from build123d import *

# Parameters (mm, degrees)
BOSS_EXTRUDE1_DEPTH      = 2.8
BOSS_EXTRUDE1_DEPTH_BACK = 2.8
ECHELLE1_SCALE           = 2
SKETCH2_R                = 1.55
CUT_EXTRUDE6_DEPTH       = 11.2


with BuildPart() as part:
    # Sketch1 → Boss-Extrude1 (new, two sides: drawn at the far end of the back side and taken through both)
    with BuildSketch(Plane.XY.offset(-BOSS_EXTRUDE1_DEPTH_BACK)):
        with BuildLine():
            Line((-33.309608541, 3.5), (9.690391459, 3.5))
            ThreePointArc((9.690391459, 3.5), (13.190391459, 0), (9.690391459, -3.5))
            Line((9.690391459, -3.5), (-33.309608541, -3.5))
            ThreePointArc((-33.309608541, -3.5), (-36.809608541, 0), (-33.309608541, 3.5))
        make_face()
    extrude(amount=BOSS_EXTRUDE1_DEPTH + BOSS_EXTRUDE1_DEPTH_BACK)


with BuildPart() as part_1:
    # Echelle1: scaled about (-11.809608541, 0, 0)
    add(part.part.scale(ECHELLE1_SCALE).moved(Location((11.809608541, 0, 0))))

    # Sketch2 → Cut-Extrude6 (cut)
    with BuildSketch(Plane.XY.offset(-5.6)):
        with Locations((-54.809608541, 0)):
            Circle(SKETCH2_R)
        with Locations((-37.609608541, 0)):
            Circle(SKETCH2_R)
        with Locations((-20.409608541, 0)):
            Circle(SKETCH2_R)
        with Locations((-3.209608541, 0)):
            Circle(SKETCH2_R)
        with Locations((13.990391459, 0)):
            Circle(SKETCH2_R)
        with Locations((31.190391459, 0)):
            Circle(SKETCH2_R)
    extrude(amount=CUT_EXTRUDE6_DEPTH, mode=Mode.SUBTRACT)


solid = part_1.part
Could you check a few things on this model? Use its own coordinates, in mm. Coordinates: 2 decimals unless noted, no trailing zeros. Order: outer loops, then holes, each group sorted by start corner. A loop starts at its lowest first (then second) coordinate and runs counter-clockwise, first axis right, second up. Notation, with made-up numbers: (23.25, 64) - (80.25, 64) arc R5 ccw to (80.25, 71) - close; hole circle Ø3 at (9.25, 65.5). An arc over 180 degrees is marked (long way). Answer in a Markdown table with one row per item. Add a question column.
(1) I need wall thicknesses on L1, parallel to Y at x = -54.5, z = 0.5; L2, parallel to X at y = -4.25, z = 2; L3, parallel to Y at x = 33, z = 4. Which ranges of each line are inside material? Lowest first, please.
(2) If we section it at B-B, the plane z = 4.75: Please give me the cut outline in (x, y).
(3) If we section it at D-D, the plane x = -3: Please give me the cut outline in (y, z), then the cut area to 3 significant figures.
(4) If we mould it in two halves opening along Y, with no side actions, what happens to faces 1 (the face through (-11, 0, 5.6)), 2 (the face through (-53.331, 0.466, -0.078)), 3 (the face through (-61.81, -0.15, -0.08))? For each: released by +Y, released by -Y, zero draft, split by the parting line, or undercut.
(5) If we section it at C-C, the plane x = -20.5: Please give me the cut outline in (y, z).
(6) If we section it at A-A, the plane y = 0: Please give me the cut outline in (x, z).
Results are:
| question | item | result |
|---|---|---|
| 1 | L1 | y = -7 to -1.52, 1.52 to 7 |
| 1 | L2 | x = -60.37 to 36.75 |
| 1 | L3 | y = -6.76 to 6.76 |
| 2 | outline | (-54.81, -7) - (31.19, -7) arc R7 ccw to (31.19, 7) - (-54.81, 7) arc R7 ccw to start; hole circle Ø3.1 at (-54.81, 0); hole circle Ø3.1 at (-37.61, 0); hole circle Ø3.1 at (-20.41, 0); hole circle Ø3.1 at (-3.21, 0); hole circle Ø3.1 at (13.99, 0); hole circle Ø3.1 at (31.19, 0) |
| 3 | outline | (-7, -5.6) - (-1.54, -5.6) - (-1.54, 5.6) - (-7, 5.6) - close; (1.54, -5.6) - (7, -5.6) - (7, 5.6) - (1.54, 5.6) - close |
| 3 | area | 122 mm2 |
| 4 | face 1 | zero draft |
| 4 | face 2 | undercut |
| 4 | face 3 | split by the parting line |
| 5 | outline | (-7, -5.6) - (-1.55, -5.6) - (-1.55, 5.6) - (-7, 5.6) - close; (1.55, -5.6) - (7, -5.6) - (7, 5.6) - (1.55, 5.6) - close |
| 6 | outline | (-61.81, -5.6) - (-56.36, -5.6) - (-56.36, 5.6) - (-61.81, 5.6) - close; (-53.26, -5.6) - (-39.16, -5.6) - (-39.16, 5.6) - (-53.26, 5.6) - close; (-36.06, -5.6) - (-21.96, -5.6) - (-21.96, 5.6) - (-36.06, 5.6) - close; (-18.86, -5.6) - (-4.76, -5.6) - (-4.76, 5.6) - (-18.86, 5.6) - close; (-1.66, -5.6) - (12.44, -5.6) - (12.44, 5.6) - (-1.66, 5.6) - close; (15.54, -5.6) - (29.64, -5.6) - (29.64, 5.6) - (15.54, 5.6) - close; (32.74, -5.6) - (38.19, -5.6) - (38.19, 5.6) - (32.74, 5.6) - close |
